Verification items for the finished model (mm, model axes). Face numbers are marked on the shaded views. A direction names the side the tool comes from. Round coordinates to 2 decimals unless told otherwise and drop trailing zeros. Write each loop counter-clockwise with the first axis right and the second up, starting at its lowest first coordinate (ties: lowest second). Pieces come first, ordered by that corner, then holes. Notation, with made-up numbers: M -10,57.5 L 48,57.5 A17 ccw 48,62.5 Z; hole C -38,-4.5 d10. An arc over 180 degrees is marked long. One line per question, with ' | ' between items. Start each with the question number.
Q1. Thickness scan on line 1 along Y through (x, z) = (12.75, -1.75); line 2 along X through (y, z) = (-108, -13); line 3 along Z through (x, y) = (3.25, -118). Record the ranges inside material, lowest first. Write a range as from..to.
Q2. Gauge pin test, flat ends, axial feed: pin 1 (2 mm diameter, centred on x = 7.5, y = -1, fed in from +Z); pin 2 (1 mm diameter, centred on y = -1, z = -14.5, fed in from -X); pin 3 (0.6 mm diameter, centred on y = -159.5, z = -14.5, fed in from +X). Record the tip position at first contact, or that the pin passes through.
Q3. Cross-section at B-B (z = -8). Record the boundary of the cut face in (x, y), then the cut area to 3 significant figures.
Q4. Tool access check on the marked faces 1 and 2. Record the directions out of +Z, -Z, +X, -X, +Y, -Y that give a thin tool (end or side, any length) a straight path to the whole face; none if there is none.
Q5. Cross-section at A-A (y = -31). Record the boundary of the cut face in (x, z), then the cut area to 3 significant figures.
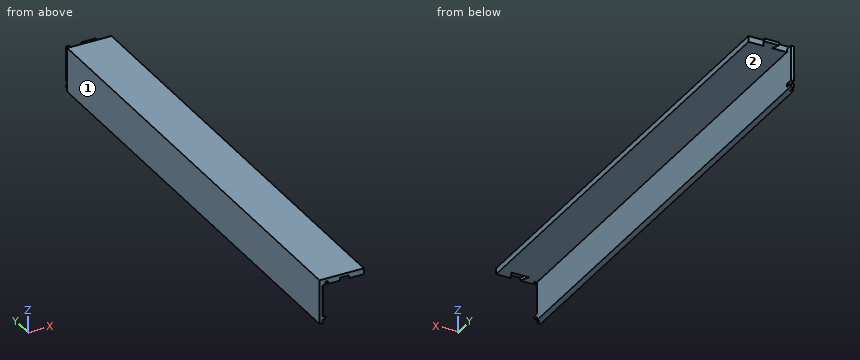
from build123d import *

# Parameters (mm, degrees)
F0_W      = 2
F0_H      = 13
F1_DEPTH  = 160
F2_W      = 1.5
F2_H      = 1.2
F2_H_2    = 10.8
F3_DEPTH  = 1
F4_W      = 0.8
F4_H      = 1.5
F5_DEPTH  = 1
F7_DEPTH  = 2
F8_W      = 2.5
F8_H      = 1.2
F9_DEPTH  = 1
F10_W     = 11
F10_H     = 2.5
F11_DEPTH = 1
F12_W     = 2.5
F12_H     = 14
F13_DEPTH = 1


with BuildPart() as f1:
    # F0 (on Front) → F1 (new body)
    with BuildSketch(Plane.XZ):
        Polygon((15, 0), (0, 0), (0, -2), (2, -2), (15, -2), align=None)
        with Locations((1, -8.5)):
            Rectangle(F0_W, F0_H)
    extrude(amount=F1_DEPTH)

    # F2 (on face) → F3 (cut)
    with BuildSketch(Plane.YZ.offset(2)):
        with Locations((-159.25, -14.4)):
            Rectangle(F2_W, F2_H)
        with Locations((-159.25, -7.4)):
            Rectangle(F2_W, F2_H_2)
    extrude(amount=-F3_DEPTH, mode=Mode.SUBTRACT)

    # F4 (on face) → F5 (cut)
    with BuildSketch(Plane(origin=(0, 0, -2), x_dir=(1, 0, 0), z_dir=(0, 0, -1))):
        Polygon((11.5, 157), (10, 160), (7, 160), (5.5, 157), align=None)
        with Locations((2.4, 159.25)):
            Rectangle(F4_W, F4_H)
    extrude(amount=-F5_DEPTH, mode=Mode.SUBTRACT)

    # F6 (on face) → F7 (cut)
    with BuildSketch(Plane(origin=(0, 0, -2), x_dir=(1, 0, 0), z_dir=(0, 0, -1))):
        Polygon((10, 2.5), (11, 0), (15, 0), (15, 2.5), align=None)
        Polygon((6, 0), (7, 2.5), (2, 2.5), (2, 0), align=None)
    extrude(amount=-F7_DEPTH, mode=Mode.SUBTRACT)

    # F8 (on face) → F9 (cut)
    with BuildSketch(Plane.YZ.offset(2)):
        with Locations((-1.25, -13.5)):
            Rectangle(F8_W, F8_H)
    extrude(amount=-F9_DEPTH, mode=Mode.SUBTRACT)

    # F10 (on face) → F11 (cut)
    with BuildSketch(Plane.XY):
        with Locations((5.5, -1.25)):
            Rectangle(F10_W, F10_H)
    extrude(amount=-F11_DEPTH, mode=Mode.SUBTRACT)

    # F12 (on face) → F13 (cut)
    with BuildSketch(Plane(origin=(0, 0, 0), x_dir=(0, -1, 0), z_dir=(-1, 0, 0))):
        with Locations((1.25, -8)):
            Rectangle(F12_W, F12_H)
    extrude(amount=-F13_DEPTH, mode=Mode.SUBTRACT)


solid = f1.part
Determined:
1) line 1: y = -160..-2.5 | line 2: x = 0..2 | line 3: z = -2..0
2) pin 1: stops at z = -1 | pin 2: stops at x = 1 | pin 3: stops at x = 1
3) outline: M 0,-160 L 1,-160 L 1,-158.5 L 2,-158.5 L 2,0 L 1,0 L 1,-2.5 L 0,-2.5 Z | area: 316 mm²
4) face 1: +Z, -Z, -X, +Y, -Y | face 2: -Z, +X, +Y, -Y
5) outline: M 0,-15 L 2,-15 L 2,-2 L 15,-2 L 15,0 L 0,0 Z | area: 56.0 mm²
